```python
from build123d import *

# Parameters (mm, degrees)
SKETCH1_R                         = 80.518
SKETCH1_R_2                       = 79.375
BOSS_EXTRUDE1_DEPTH               = 974.725
F_10_0_1935_DIAMETER_HOLE1_REACH  = 993.214
F_10_0_1935_DIAMETER_HOLE1_BORE_R = 2.45745
CIRPATTERN1_COUNT                 = 6


with BuildPart() as part:
    # Sketch1 → Boss-Extrude1 (new body)
    with BuildSketch(Plane.XY):
        with Locations(Location((0, 0, 0), (0, 0, 180))):
            Circle(SKETCH1_R)
        with Locations(Location((0, 0, 0), (0, 0, 180))):
            Circle(SKETCH1_R_2, mode=Mode.SUBTRACT)
    extrude(amount=BOSS_EXTRUDE1_DEPTH)

    # #10 (0.1935) Diameter Hole1 bore → #10 (0.1935) Diameter Hole1 (cut, up to next)
    with BuildSketch(Plane(origin=(0, 80.518, 0), x_dir=(1, 0, 0), z_dir=(0, 1, 0)), mode=Mode.PRIVATE) as f_10_0_1935_diameter_hole1_sk1:
        with Locations((0, -79.375)):
            Circle(F_10_0_1935_DIAMETER_HOLE1_BORE_R)
    f_10_0_1935_diameter_hole1_tool1 = extrude(f_10_0_1935_diameter_hole1_sk1.sketch, amount=-F_10_0_1935_DIAMETER_HOLE1_REACH, mode=Mode.PRIVATE) & part.part
    f_10_0_1935_diameter_hole1 = f_10_0_1935_diameter_hole1_tool1.solids().sort_by_distance((0, 80.518, 79.375))[0]
    add(f_10_0_1935_diameter_hole1, mode=Mode.SUBTRACT)

    # CirPattern1: #10 (0.1935) Diameter Hole1 ×6 about axis
    cirpattern1_axis = Axis((0, 0, 0), (0, 0, 1))
    for i in range(1, CIRPATTERN1_COUNT):
        add(f_10_0_1935_diameter_hole1.rotate(cirpattern1_axis, i * 360 / CIRPATTERN1_COUNT), mode=Mode.SUBTRACT)


solid = part.part
```
Geometry: final body of the model. Coordinates: model frame, mm. Give positions to 0.01 mm unless a question says otherwise; leave off trailing zeros. Order: outer loops, then holes, each group sorted by start corner. A loop starts at its lowest first (then second) coordinate and runs counter-clockwise, first axis right, second up. Notation, with made-up numbers: (75.5, -18) -> (79.5, -18) arc R18 cw to (79.5, -6) -> close; hole circle Ø10 at (-22, 78). An arc over 180 degrees is marked (long way). Write each question's results on one line, items separated by ' | '. Start each with the question number.
1) Draft query along X for faces 1 (the cylindrical face through (-37.154, 71.433, 480.539)), 2 (the flat face through (-59.3, 53.3, 0)), 3 (the cylindrical face through (-75.71, -23.84, 480.54)). Return one class per face: pulls with the +X half, pulls with the -X half, needs draft (parallel to the pull), parting line crosses it, or undercut.
2) Section C-C (z = 479). Return loops of the section in (x, y) (3 decimals), then the cut area to 3 significant figures.
3) Line query: line 1 (Y direction, x = 0, z = 734) (3 decimals); line 2 (Z direction, x = 0, y = 80.35) (3 decimals); line 3 (Y direction, x = -54, z = 514.5). Output: solid intervals per line, ascending. Write a range as from..to.
4) Section B-B (x = 12). Return loops of the section in (y, z) (3 decimals).
5) Section A-A (y = 0). Return loops of the section in (x, z) (3 decimals), then the cut area to 3 significant figures.
6) First-contact query: pin 1 (2 mm diameter, centred on x = -57, z = 562, fed in from -Y); pin 2 (4 mm diameter, centred on y = 43.5, z = 378, fed in from -X); pin 3 (4.5 mm diameter, centred on x = 0, z = 79.375, fed in from -Y); pin 4 (1 mm diameter, centred on y = 27, z = 859, fed in from -X). Flat tips, straight axial feed; report the tip coordinate or a pass-through.
Calculated:
1) face 1: parting line crosses it | face 2: needs draft | face 3: undercut
2) outline: circle Ø161.036 at (0, 0); hole circle Ø158.75 at (0, 0) | area: 574 mm2
3) line 1: -80.518..-79.375, 79.375..80.518 | line 2: 0..76.918, 81.832..974.725 | line 3: -59.73..-58.18, 58.18..59.73
4) outline: (-79.619, 0) -> (-78.463, 0) -> (-78.463, 974.725) -> (-79.619, 974.725) -> close; (78.463, 0) -> (79.619, 0) -> (79.619, 974.725) -> (78.463, 974.725) -> close
5) outline: (-80.518, 0) -> (-79.375, 0) -> (-79.375, 974.725) -> (-80.518, 974.725) -> close; (79.375, 0) -> (80.518, 0) -> (80.518, 974.725) -> (79.375, 974.725) -> close | area: 2,230 mm2
6) pin 1: y = -57.85 | pin 2: x = -69 | pin 3: through | pin 4: x = -76.03
